Check sheet for the modelled part. Datum: model origin and axes. Units: mm. A direction names the side the tool comes from. Give positions to 0.01 mm unless a question says otherwise; leave off trailing zeros. Order: outer loops, then holes, each group sorted by start corner. A loop starts at its lowest first (then second) coordinate and runs counter-clockwise, first axis right, second up.
Autodesk Inventor part; units mm, degrees
ref_plane "YZ Plane" through (0, 0, 0) normal (1, 0, 0) x (0, 1, 0)
ref_plane "XZ Plane" through (0, 0, 0) normal (0, 1, 0) x (-1, 0, 0)
ref_plane "XY Plane" through (0, 0, 0) normal (0, 0, 1) x (1, 0, 0)
sketch "Sketch1" plane through (0, 0, 0) normal (0, 0, 1) x (1, 0, 0)
  line L0 (-17.5, -12.5) -> (17.5, -12.5)
  line L1 (17.5, -12.5) -> (17.5, 12.5)
  line L2 (17.5, 12.5) -> (-17.5, 12.5)
  line L3 (-17.5, 12.5) -> (-17.5, -12.5)
  line L4 (-17.5, -12.5) -> (17.5, 12.5) construction
  line L5 (17.5, -12.5) -> (-17.5, 12.5) construction
  point P0 (0, 0)
  dimension "d0" = 35
  dimension "d1" = 25
extrude "Extrusion1" add sketch "Sketch1" along normal blind 130
sketch "Sketch2" plane through (-17.5, -12.5, 0) normal (0, -1, 0) x (1, 0, 0)
  line L0 (2, 115) -> (0, 115)
  line L1 (0, 115) -> (0, 130)
  line L2 (0, 130) -> (2, 130)
  line L3 (2, 130) -> (2, 115)
  line L4 (0, 0) -> (0, 130)
  line L5 (0, 130) -> (35, 130)
  point P0 (17.5, 0)
  dimension "d4" = 2
  dimension "d5" = 15
extrude "Extrusion2" cut sketch "Sketch2" against normal through all
sketch "Sketch3" plane through (-17.5, -12.5, 0) normal (0, -1, 0) x (1, 0, 0)
  line L0 (2, 130) -> (35, 130)
  line L1 (35, 0) -> (35, 130)
  line L2 (0, 0) -> (35, 0)
  point P0 (17.5, 0)
  point P1 (20, 105)
  point P2 (20, 25)
  dimension "d8" = 25
  dimension "d9" = 15
  dimension "d10" = 25
hole "Hole1" at (2.5, -12.5, 105) at (2.5, -12.5, 25) direction (0, 1, 0) diameter 5.5 end through all counterbore diameter 15 counterbore depth 9
properties part number "Distanzblock_rechts" material "Aluminum 6061"
(1) Cross-section at A-A on z = 105. Enter the section's corners in (x, y), then the cut area to 3 significant figures.
Response values:
outline: (-17.5, -12.5) - (-5, -12.5) - (-5, -3.5) - (-0.25, -3.5) - (-0.25, 12.5) - (-17.5, 12.5) - close; (5.25, -3.5) - (10, -3.5) - (10, -12.5) - (17.5, -12.5) - (17.5, 12.5) - (5.25, 12.5) - close
area: 652 mm2
(2) Cross-section at D-D on z = 119.5. Enter the section's corners in (x, y).
Response values:
outline: (-15.5, -12.5) - (17.5, -12.5) - (17.5, 12.5) - (-15.5, 12.5) - close
(3) Material ranges on L1, parallel to Z at x = 2.5, y = -9; L2, parallel to Z at x = 2.5, y = 3.5; L3, parallel to X at y = 2.5, z = 105, recorded low to high.
Response values:
L1: z = 0 to 17.5, 32.5 to 97.5, 112.5 to 130
L2: z = 0 to 22.25, 27.75 to 102.25, 107.75 to 130
L3: x = -17.5 to -0.25, 5.25 to 17.5
(4) Cross-section at B-B on x = 2.5. Enter the section's corners in (y, z).
Response values:
outline: (-12.5, 0) - (12.5, 0) - (12.5, 22.25) - (-3.5, 22.25) - (-3.5, 17.5) - (-12.5, 17.5) - close; (-12.5, 32.5) - (-3.5, 32.5) - (-3.5, 27.75) - (12.5, 27.75) - (12.5, 102.25) - (-3.5, 102.25) - (-3.5, 97.5) - (-12.5, 97.5) - close; (-12.5, 112.5) - (-3.5, 112.5) - (-3.5, 107.75) - (12.5, 107.75) - (12.5, 130) - (-12.5, 130) - close
(5) Set-up check for faces 4 (the face through (2, -3.5, 22)), 5 (the face through (-15.5, 0, 123)), 6 (the face through (17.5, 0, 64)): record each of +Z, -Z, +X, -X, +Y, -Y from which the full face is reachable in a straight line by a thin tool's end or side.
Response values:
face 4: -Y
face 5: +Z, -X, +Y, -Y
face 6: +Z, -Z, +X, +Y, -Y
(6) Cross-section at C-C on y = 6.75. Enter the section's corners in (x, z).
Response values:
outline: (-17.5, 0) - (17.5, 0) - (17.5, 130) - (-15.5, 130) - (-15.5, 115) - (-17.5, 115) - close; hole circle Ø5.5 at (2.5, 25); hole circle Ø5.5 at (2.5, 105)
(7) Gauge pin test, flat ends, axial feed: pin 1 Ø17 at (x, z) = (2.5, 105) entering from -Y; pin 2 Ø3.5 at (x, z) = (2.5, 25) entering from -Y; pin 3 Ø12 at (x, z) = (2.5, 25) entering from -Y. Record the tip position at first contact, or that the pin passes through.
Response values:
pin 1: stops at y = -12.5
pin 2: passes through
pin 3: stops at y = -3.5
(8) Release check for a two-part mould opening along Z. For faces 1 (the face through (0, 0, 0)), 2 (the face through (-17.5, 0, 57)), 3 (the face through (2.379, 4.612, 27.747)) record: released by +Z, released by -Z, zero draft, split by the parting line, or undercut.
Response values:
face 1: released by -Z
face 2: zero draft
face 3: undercut
